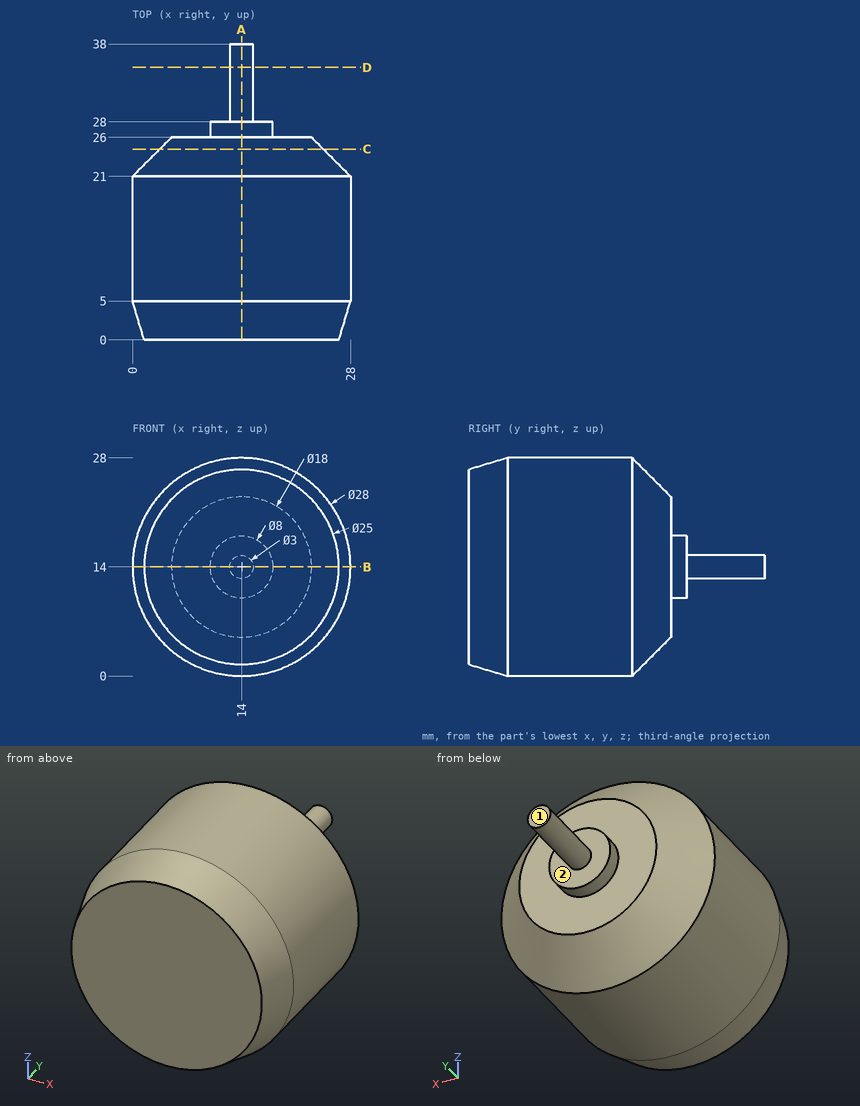
Could you check a few things on this drawing? It's one solid part, dimensions in mm from its lowest x, y, z. A direction names the side the tool comes from. Give positions to 0.01 mm unless a question says otherwise; leave off trailing zeros. Write each loop counter-clockwise with the first axis right and the second up, starting at its lowest first coordinate (ties: lowest second). Pieces come first, ordered by that corner, then holes. Notation, with made-up numbers: (13.5, 66) -> (50.5, 66) arc R19 cw to (50.5, 98) -> close; hole circle Ø11 at (56.5, 38.25). An arc over 180 degrees is marked (long way). Answer as CSV lines item,"result". Start each with the question number.
(1) Please list where these lines run through material, in increasing order: line 1 (Y direction, x = 12, z = 13.5); line 2 (Y direction, x = 16, z = 8.5); line 3 (Z direction, x = 14.5, y = 12).
(2) If we section it at D-D, the plane y = 35: Write out the boundary of the cut face in (x, z).
(3) If we section it at A-A, the plane x = 14: Write out the boundary of the cut face in (y, z), and give its area (4 significant figures).
(4) I'm going to push flat-ended pins straight in: pin 1 Ø4 at (x, z) = (16.5, 7.5) entering from -Y; pin 2 Ø8 at (y, z) = (16, 23.5) entering from -X; pin 3 Ø1 at (x, y) = (23, 8.5) entering from +Z; pin 4 Ø10 at (x, y) = (22, 14.5) entering from -Z. Where does each tip first touch, or does it pass through?
(5) Which directions (+Z, -Z, +X, -X, +Y, -Y) give clear straight access to the entire face, cutting with the end or side of a thin tool? Please do the marked faces 1 and 2.
(6) If we section it at B-B, the plane z = 14: Write out the boundary of the cut face in (x, y).
(7) If we section it at C-C, the plane y = 24.5: Write out the boundary of the cut face in (x, z).
Answer list:
1,line 1,"0 to 28"
1,line 2,"0 to 26"
1,line 3,"0.01 to 27.99"
2,outline,"circle Ø3 at (14, 14)"
3,outline,"(0, 1.5) -> (5, 0) -> (21, 0) -> (26, 5) -> (26, 10) -> (28, 10) -> (28, 12.5) -> (38, 12.5) -> (38, 15.5) -> (28, 15.5) -> (28, 18) -> (26, 18) -> (26, 23) -> (21, 28) -> (5, 28) -> (0, 26.5) -> close"
3,area,"741.5 mm^2"
4,pin 1,"y = 0"
4,pin 2,"x = 1.13"
4,pin 3,"z = 25.12"
4,pin 4,"z = 0.33"
5,face 1,"+Z, -Z, +X, -X, +Y"
5,face 2,"+Y"
6,outline,"(0, 5) -> (1.5, 0) -> (26.5, 0) -> (28, 5) -> (28, 21) -> (23, 26) -> (18, 26) -> (18, 28) -> (15.5, 28) -> (15.5, 38) -> (12.5, 38) -> (12.5, 28) -> (10, 28) -> (10, 26) -> (5, 26) -> (0, 21) -> close"
7,outline,"circle Ø21 at (14, 14)"
